Check sheet for the drawn part. Datum: minimum x, y, z corner. Units: mm. A direction names the side the tool comes from. Give positions to 0.01 mm unless a question says otherwise; leave off trailing zeros. Order: outer loops, then holes, each group sorted by start corner. A loop starts at its lowest first (then second) coordinate and runs counter-clockwise, first axis right, second up.
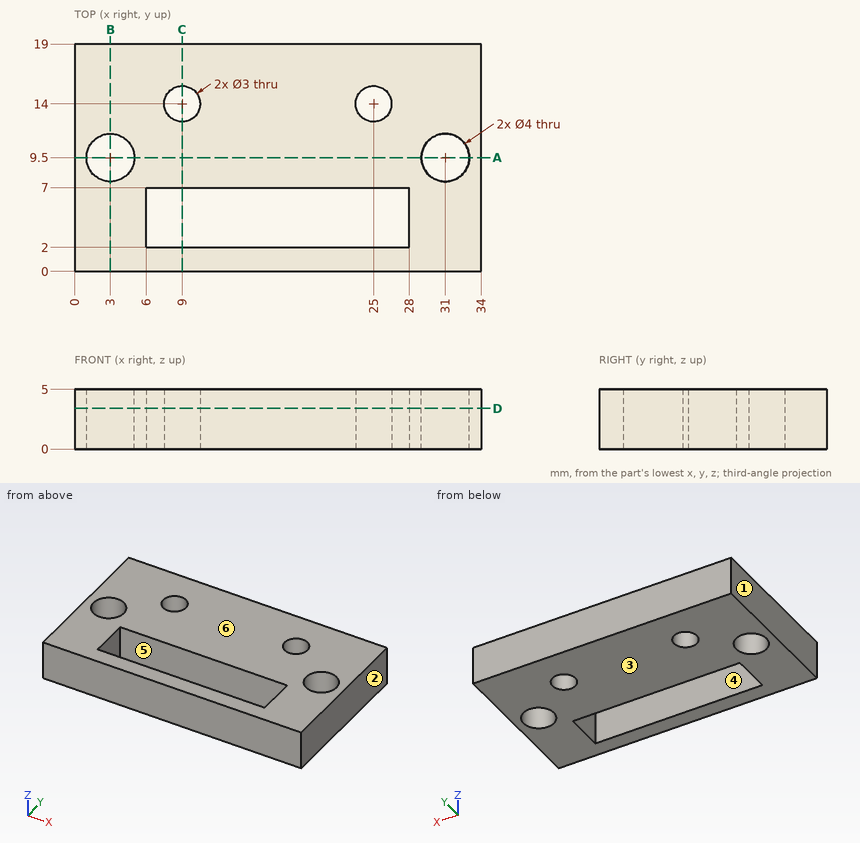
Item 1: Draft check along X on the marked faces 1, 2, 3 and 4. Enter one of: released by +X, released by -X, zero draft, split by the parting line, or undercut.
Reported:
face 1: released by -X
face 2: released by +X
face 3: zero draft
face 4: undercut
Item 2: Sectioned sample at A-A (y = 9.5). Enter the section's corners in (x, z), and give its area (3 significant figures).
Reported:
outline: (0, 0) - (1, 0) - (1, 5) - (0, 5) - close; (5, 0) - (29, 0) - (29, 5) - (5, 5) - close; (33, 0) - (34, 0) - (34, 5) - (33, 5) - close
area: 130 mm2
Item 3: Sectioned sample at D-D (z = 3.4). Enter the section's corners in (x, y).
Reported:
outline: (0, 0) - (34, 0) - (34, 19) - (0, 19) - close; hole circle Ø4 at (3, 9.5); hole (6, 2) - (28, 2) - (28, 7) - (6, 7) - close; hole circle Ø3 at (9, 14); hole circle Ø3 at (25, 14); hole circle Ø4 at (31, 9.5)
Item 4: Sectioned sample at C-C (x = 9). Enter the section's corners in (y, z), and give its area (3 significant figures).
Reported:
outline: (0, 0) - (2, 0) - (2, 5) - (0, 5) - close; (7, 0) - (12.5, 0) - (12.5, 5) - (7, 5) - close; (15.5, 0) - (19, 0) - (19, 5) - (15.5, 5) - close
area: 55.0 mm2
Item 5: Set-up check for the marked faces 5 and 6: record each of +Z, -Z, +X, -X, +Y, -Y from which the full face is reachable in a straight line by a thin tool's end or side.
Reported:
face 5: +Z, -Z
face 6: +Z, +X, -X, +Y, -Y
Item 6: Sectioned sample at B-B (x = 3). Enter the section's corners in (y, z), and give its area (3 significant figures).
Reported:
outline: (0, 0) - (7.5, 0) - (7.5, 5) - (0, 5) - close; (11.5, 0) - (19, 0) - (19, 5) - (11.5, 5) - close
area: 75.0 mm2
Item 7: Scan lines: L1, parallel to Y at x = 9, z = 3.1; L2, parallel to Y at x = 3, z = 1.35; L3, parallel to X at y = 4.75, z = 3.3. Record each from-to range of solid material in increasing order.
Reported:
L1: y = 0 to 2, 7 to 12.5, 15.5 to 19
L2: y = 0 to 7.5, 11.5 to 19
L3: x = 0 to 6, 28 to 34
